```python
from build123d import *

# Parameters (mm, degrees)
CROQUIS2_W              = 100
CROQUIS2_H              = 50
SALIENTE_EXTRUIR1_DEPTH = 30
CORTAR_EXTRUIR1_DEPTH   = 15
CORTAR_EXTRUIR2_DEPTH   = 20
CORTAR_EXTRUIR3_DEPTH   = 165.121269


with BuildPart() as part:
    # Croquis2 → Saliente-Extruir1 (new, symmetric)
    with BuildSketch(Plane.XY):
        with Locations((50, 25)):
            Rectangle(CROQUIS2_W, CROQUIS2_H)
    extrude(amount=SALIENTE_EXTRUIR1_DEPTH, both=True)

    # Croquis3 → Cortar-Extruir1 (cut)
    with BuildSketch(Plane.ZY):
        Polygon((30, 50), (30, 40), (10, 50), align=None)
    cortar_extruir1 = extrude(amount=-CORTAR_EXTRUIR1_DEPTH, mode=Mode.SUBTRACT)

    # Croquis4 → Cortar-Extruir2 (cut)
    with BuildSketch(Plane.XZ):
        Polygon((100, 0), (90, 30), (100, 30), align=None)
    cortar_extruir2 = extrude(amount=-CORTAR_EXTRUIR2_DEPTH, mode=Mode.SUBTRACT)

    # Croquis6 → Cortar-Extruir3 (cut, through all, along a direction that is not the sketch's normal)
    with BuildSketch(Plane(origin=(0, 50, 0), x_dir=(1, 0, 0), z_dir=(0, 1, 0))):
        Polygon((100, 0), (70, 0), (40, -30), (100, -30), align=None)
    cortar_extruir3 = extrude(amount=-CORTAR_EXTRUIR3_DEPTH, dir=(-0.7071067811865475, 0.7071067811865476, 0), mode=Mode.SUBTRACT)

    # Simetría1: Cortar-Extruir1, Cortar-Extruir2, Cortar-Extruir3 across plane
    add(cortar_extruir1.mirror(Plane.XY), mode=Mode.SUBTRACT)
    add(cortar_extruir2.mirror(Plane.XY), mode=Mode.SUBTRACT)
    add(cortar_extruir3.mirror(Plane.XY), mode=Mode.SUBTRACT)


solid = part.part
```
Design review of the part built by this model. Coordinates are the model's own, in mm. A direction names the side the tool comes from. Round coordinates to 2 decimals unless told otherwise and drop trailing zeros. Order: outer loops, then holes, each group sorted by start corner. A loop starts at its lowest first (then second) coordinate and runs counter-clockwise, first axis right, second up. Notation, with made-up numbers: (-17.5, -29.75) - (30.5, -29.75) arc R8 ccw to (30.5, -25.75) - close; hole circle Ø7 at (71.5, 82). An arc over 180 degrees is marked (long way). One line per question, with ' | ' between items.
Item 1: Take a section at D-D, the plane y = 42.5. Write out the cut boundary in (x, z), then the cut area to 3 significant figures.
Checks:
outline: (0, -25) - (15, -25) - (15, -30) - (47.5, -30) - (77.5, 0) - (47.5, 30) - (15, 30) - (15, 25) - (0, 25) - close | area: 3,600 mm²
Item 2: Take a section at C-C, the plane z = -7.5. Write out the cut boundary in (x, y), then the cut area to 3 significant figures.
Checks:
outline: (0, 0) - (97.5, 0) - (97.5, 15) - (62.5, 50) - (0, 50) - close | area: 4,260 mm²
Item 3: Take a section at B-B, the plane x = 60.5. Write out the cut boundary in (y, z).
Checks:
outline: (0, -30) - (29.5, -30) - (50, -9.5) - (50, 9.5) - (29.5, 30) - (0, 30) - close
Item 4: Wall thickness on line 1 (Y direction, x = 83, z = 7); line 2 (X direction, y = 27.5, z = 6); line 3 (X direction, y = 47, z = -28): over which ranges is each line inside the solid? List them lowest first. Write a range as [from, to].
Checks:
line 1: [0, 30] | line 2: [0, 86.5] | line 3: [15, 45]
Item 5: For P1, Ø1, axis at x = 62, z = 11.5, coming from the +Y side; P2, Ø1.5, axis at y = 23.5, z = 4.5, coming from the -X side; P3, Ø1, axis at x = 83, y = 33.5, coming from the +Z side; P4, Ø12, axis at x = 87, y = 30.5, coming from the +Z side, all flat-tipped, find the tip position at first contact; note any pin that passes through.
Checks:
P1: y = 47.21 | P2: x = 0 | P3: z = 4.21 | P4: z = 10.99
Item 6: Take a section at A-A, the plane y = 18. Write out the cut boundary in (x, z).
Checks:
outline: (0, -30) - (72, -30) - (99, -3) - (100, 0) - (99, 3) - (72, 30) - (0, 30) - close
Item 7: Machinability: for faces 1 (the face through (7, 45, 20)), 2 (the face through (96.18, 7.64, 11.46)), 3 (the face through (7, 45, -20)), which of the approach directions +Z, -Z, +X, -X, +Y, -Y give a long, thin tool a straight path to every point of the face, cutting with its end or side? Answer none if there is none.
Checks:
face 1: +Z, -X, +Y | face 2: +Z, +X, +Y, -Y | face 3: -Z, -X, +Y
